Work out the finished part from the listing and answer in its coordinate system (mm). Face numbers are marked on the shaded views. A direction names the side the tool comes from. Coordinates: 2 decimals unless noted, no trailing zeros. Order: outer loops, then holes, each group sorted by start corner. A loop starts at its lowest first (then second) coordinate and runs counter-clockwise, first axis right, second up. Notation, with made-up numbers: M 73,65.5 L 101,65.5 A5 ccw 101,70.5 Z; hole C 64.25,70 d11. An arc over 180 degrees is marked long. Answer in a Markdown table with one row per item. Add a question column.
Item 1: Which of the six approach directions +Z, -Z, +X, -X, +Y, -Y give full straight-line access (tool end or side, diameter ignored) to the marked faces 1 and 2?
Item 2: The part is cut by section D-D (x = -10.25). Write down the section's boundary in (y, z).
Item 3: Consider line 1 (Z direction, x = 0, y = 0.75); line 2 (Z direction, x = 0, y = 7.5); line 3 (X direction, y = -5.5, z = -37). Determine where each line is inside the solid, lowest interval first. Write a range as from..to.
Item 4: The part is cut by section A-A (x = 0). Write down the section's boundary in (y, z).
Item 5: Flat-ended cylindrical pins translate along their axes: pin 1 Ø1.5 at (y, z) = (8.5, 5.5) entering from -X; pin 2 Ø10 at (x, y) = (1, 6) entering from +Z; pin 3 Ø8 at (y, z) = (8, -25.5) entering from -X; pin 4 Ø1.5 at (y, z) = (-7.5, -42.5) entering from -X. Find the tip coordinate at first contact, or state that the pin passes through.
Item 6: The part is cut by section B-B (z = 15.5). Write down the section's boundary in (x, y).
Item 7: The part is cut by section C-C (y = 0). Write down the section's boundary in (x, z), then the cut area to 3 significant figures.
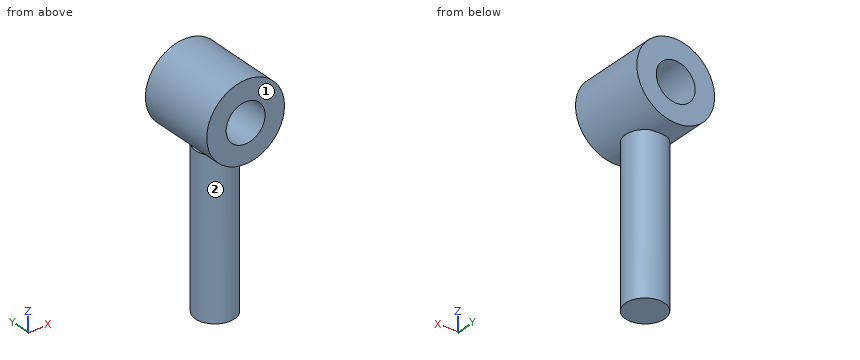
from build123d import *

# Parameters (mm, degrees)
F0_R     = 6.35
F1_DEPTH = 50.8
F2_R     = 12.7
F3_DEPTH = 12.7
F4_R     = 6.35
F5_DEPTH = 12.7


with BuildPart() as f1:
    # F0 (on Top) → F1 (new body)
    with BuildSketch(Plane.XY):
        Circle(F0_R)
    extrude(amount=-F1_DEPTH)

    # F2 (on Front) → F3 (join, symmetric)
    with BuildSketch(Plane.XZ):
        with Locations((0, 12.382501)):
            Circle(F2_R)
    extrude(amount=F3_DEPTH, both=True)

    # F4 (on Front) → F5 (cut, symmetric)
    with BuildSketch(Plane.XZ):
        with Locations((0, 12.110357)):
            Circle(F4_R)
    extrude(amount=F5_DEPTH, both=True, mode=Mode.SUBTRACT)


solid = f1.part
Reply:
| question | item | result |
|---|---|---|
| 1 | face 1 | +Z, -Z, +X, -X, -Y |
| 1 | face 2 | -Z |
| 2 | outline | M -12.7,4.88 L 12.7,4.88 L 12.7,19.88 L -12.7,19.88 Z |
| 3 | line 1 | z = -50.8..5.76, 18.46..25.08 |
| 3 | line 2 | z = -0.32..5.76, 18.46..25.08 |
| 3 | line 3 | x = -3.17..3.17 |
| 4 | outline | M -12.7,-0.32 L -6.35,-0.32 L -6.35,-50.8 L 6.35,-50.8 L 6.35,-0.32 L 12.7,-0.32 L 12.7,5.76 L -12.7,5.76 Z; M -12.7,18.46 L 12.7,18.46 L 12.7,25.08 L -12.7,25.08 Z |
| 5 | pin 1 | stops at x = -11.12 |
| 5 | pin 2 | stops at z = 25.08 |
| 5 | pin 3 | stops at x = -4.93 |
| 5 | pin 4 | passes through |
| 6 | outline | M -12.31,-12.7 L -5.37,-12.7 L -5.37,12.7 L -12.31,12.7 Z; M 5.37,-12.7 L 12.31,-12.7 L 12.31,12.7 L 5.37,12.7 Z |
| 7 | outline | M -6.35,-50.8 L 6.35,-50.8 L 6.35,0 L 2.82,0 A12.7 ccw long -2.82,0 L -6.35,0 Z; hole C 0,12.11 d12.7 |
| 7 | area | 1,020 mm2 |
